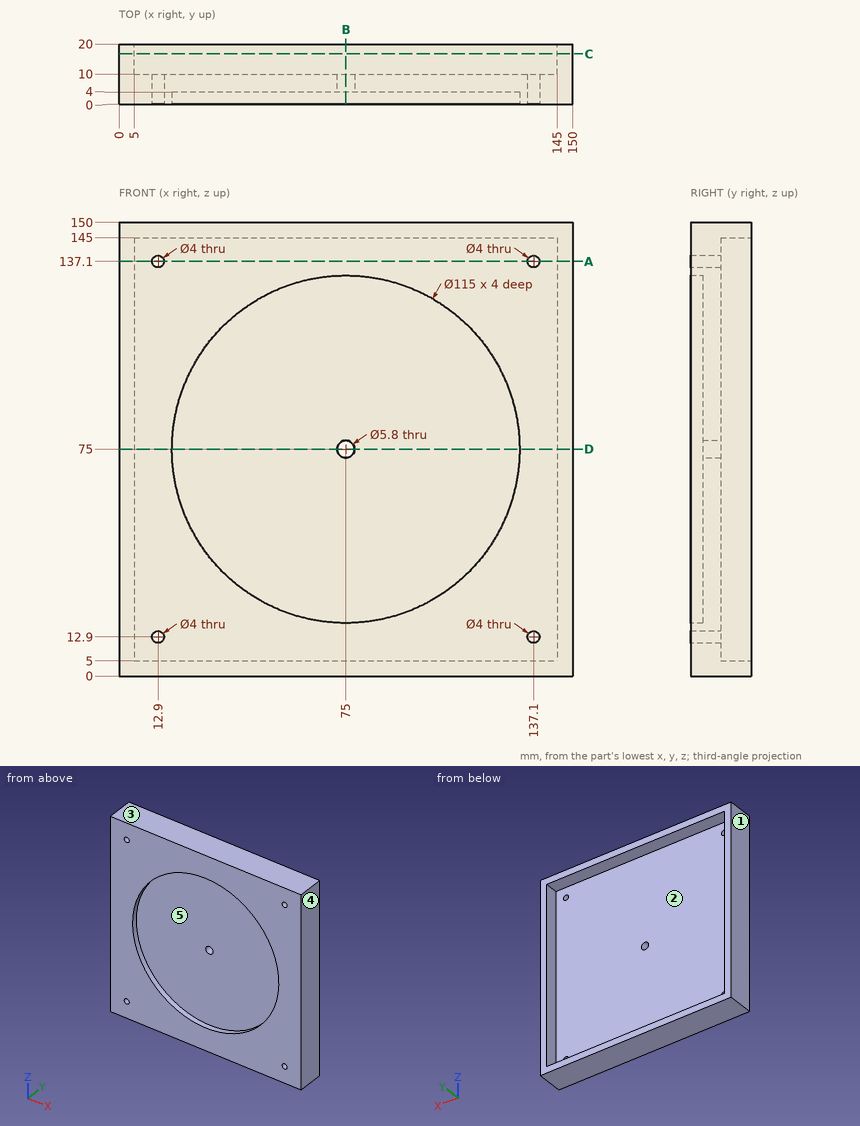
Check sheet for the drawn part. Datum: minimum x, y, z corner. Units: mm. A direction names the side the tool comes from. Round coordinates to 2 decimals unless told otherwise and drop trailing zeros. Order: outer loops, then holes, each group sorted by start corner. A loop starts at its lowest first (then second) coordinate and runs counter-clockwise, first axis right, second up.
(1) Cross-section at B-B, the plane x = 75. Enter the section's corners in (y, z).
(2) Draft check along Z on the marked faces 1, 2 and 3. Enter one of: pulls with the +Z half, pulls with the -Z half, needs draft (parallel to the pull), parting line crosses it, or undercut.
(3) Cross-section at A-A, the plane z = 137.1. Enter the section's corners in (x, y).
(4) Go/stop test with flat-tipped pins: P1, Ø2, axis at x = 80, z = 128.5, coming from the -Y side; P2, Ø3, axis at x = 122.5, z = 52.5, coming from the +Y side. Record where each tip stops, or that it passes through.
(5) Scan lines: probe 1 along X at (y, z) = (7.25, 12.9); probe 2 along X at (y, z) = (6.3, 75). Record each from-to range of solid material in increasing order.
(6) Cross-section at D-D, the plane z = 75. Enter the section's corners in (x, y), and give its area (3 significant figures).
(7) Access from +Z, -Z, +X, -X, +Y, -Y to the whole of each face (thin tool, end or side, straight path). Record for the marked faces 4 and 5.
(8) Cross-section at C-C, the plane y = 16.75. Enter the section's corners in (x, z), and give its area (3 significant figures).
Check sheet entries:
1. outline: (0, 0) - (20, 0) - (20, 5) - (10, 5) - (10, 72.1) - (4, 72.1) - (4, 17.5) - (0, 17.5) - close; (0, 132.5) - (4, 132.5) - (4, 77.9) - (10, 77.9) - (10, 145) - (20, 145) - (20, 150) - (0, 150) - close
2. face 1: needs draft
2. face 2: undercut
2. face 3: pulls with the +Z half
3. outline: (0, 0) - (10.9, 0) - (10.9, 10) - (5, 10) - (5, 20) - (0, 20) - close; (14.9, 0) - (135.1, 0) - (135.1, 10) - (14.9, 10) - close; (139.1, 0) - (150, 0) - (150, 20) - (145, 20) - (145, 10) - (139.1, 10) - close
4. P1: stops at y = 4
4. P2: stops at y = 10
5. probe 1: x = 0 to 10.9, 14.9 to 135.1, 139.1 to 150
5. probe 2: x = 0 to 72.1, 77.9 to 150
6. outline: (0, 0) - (17.5, 0) - (17.5, 4) - (72.1, 4) - (72.1, 10) - (5, 10) - (5, 20) - (0, 20) - close; (77.9, 4) - (132.5, 4) - (132.5, 0) - (150, 0) - (150, 20) - (145, 20) - (145, 10) - (77.9, 10) - close
6. area: 1,110 mm2
7. face 4: +Z, -Z, +X, +Y, -Y
7. face 5: -Y
8. outline: (0, 0) - (150, 0) - (150, 150) - (0, 150) - close; hole (5, 5) - (145, 5) - (145, 145) - (5, 145) - close
8. area: 2,900 mm2
